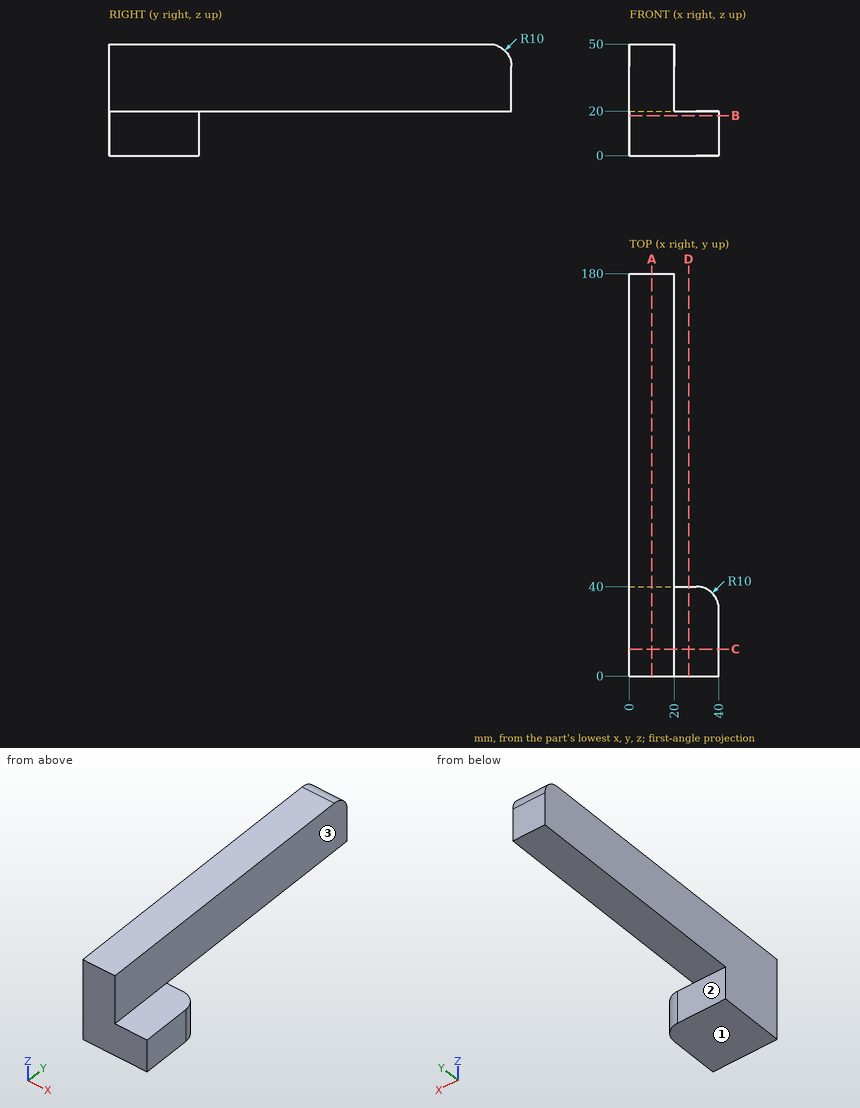
The figure shows three views and two pictorial views of one solid part (mm, origin at its lowest corner). Answer the questions. A direction names the side the tool comes from. Round coordinates to 2 decimals unless told otherwise and drop trailing zeros. Order: outer loops, then holes, each group sorted by start corner. A loop starts at its lowest first (then second) coordinate and runs counter-clockwise, first axis right, second up. Notation, with made-up numbers: M 64.25,10 L 81.25,10 A28 ccw 81.25,31 Z; hole C -36.75,3.5 d2. An arc over 180 degrees is marked long. Put each result on its own line as item: value. Start each with the question number.
Q1. Section B-B, the plane z = 18 is taken. Write down the section's boundary in (x, y), and give its area (3 significant figures).
Q2. A tool of negligible diameter and unlimited length cuts with its end or side. For the marked faces 1, 2 and 3, from which of +Z, -Z, +X, -X, +Y, -Y can it reach the whole face along a straight path? Write none if from no direction.
Q3. Section A-A, the plane x = 10 is taken. Write down the section's boundary in (y, z).
Q4. Section D-D, the plane x = 26.5 is taken. Write down the section's boundary in (y, z), and give its area (3 significant figures).
Q5. Section C-C, the plane y = 12 is taken. Write down the section's boundary in (x, z).
Q6. Straight lines are drawn through the part: L1, parallel to Z at x = 10, y = 85; L2, parallel to X at y = 57.5, z = 37. For each, find the intervals that lie inside material, in ascending order. Write a range as [from, to].
Q7. Flat-ended cylindrical pins translate along their axes: pin 1 (1.5 mm diameter, centred on y = 140.5, z = 34.5, fed in from +X); pin 2 (16 mm diameter, centred on x = 17.5, z = 10.5, fed in from +Y); pin 3 (4 mm diameter, centred on x = 9, z = 42.5, fed in from +Y); pin 4 (5 mm diameter, centred on y = 112.5, z = 33.5, fed in from -X). Find the tip coordinate at first contact, or state that the pin passes through.
Findings below:
1. outline: M 0,0 L 40,0 L 40,30 A10 ccw 30,40 L 0,40 Z
1. area: 1,580 mm^2
2. face 1: -Z, +X, -X, +Y, -Y
2. face 2: -Z, +X, -X, +Y
2. face 3: +Z, +X, +Y, -Y
3. outline: M 0,0 L 40,0 L 40,20 L 180,20 L 180,40 A10 ccw 170,50 L 0,50 Z
4. outline: M 0,0 L 40,0 L 40,20 L 0,20 Z
4. area: 800 mm^2
5. outline: M 0,0 L 40,0 L 40,20 L 20,20 L 20,50 L 0,50 Z
6. L1: z = [20, 50]
6. L2: x = [0, 20]
7. pin 1: stops at x = 20
7. pin 2: stops at y = 40
7. pin 3: stops at y = 179.99
7. pin 4: stops at x = 0
